Work out the finished part from the listing and answer in its coordinate system (mm). Round coordinates to 2 decimals unless told otherwise and drop trailing zeros. Order: outer loops, then holes, each group sorted by start corner. A loop starts at its lowest first (then second) coordinate and runs counter-clockwise, first axis right, second up. Notation, with made-up numbers: (26.5, 30) - (63.5, 30) arc R22 ccw to (63.5, 64) - close; hole circle Ø1 at (-3, -36.75). An arc over 180 degrees is marked (long way). Answer in a Markdown table with one row per item.
from build123d import *

# Parameters (mm, degrees)
BOSS_EXTRUDE1_DEPTH      = 39.6875
SKETCH2_R                = 1.4351
CUT_EXTRUDE1_DEPTH       = 42.03119412
F_5_16_24_TAPPED_HOLE1_D = 6.9088


with BuildPart() as part:
    # Sketch1 → Boss-Extrude1 (new body)
    with BuildSketch(Plane.XY):
        Polygon((0, 0), (9.9187, 0), (6.7437, -3.175), (0, -3.175), align=None)
    extrude(amount=BOSS_EXTRUDE1_DEPTH)

    # Mirror1: part across plane


with BuildPart() as part_1:
    add(part.part)
    add(part.part.mirror(Plane(origin=(0, -3.175, 39.6875), x_dir=(0, 0, 1), z_dir=(1, 0, 0))))

    # Sketch2 → Cut-Extrude1 (cut, through all)
    with BuildSketch(Plane(origin=(0, 0, 0), x_dir=(1, 0, 0), z_dir=(0, 1, 0))):
        with Locations(Location((0, -36.5125, 0), (0, 0, 180))):
            Circle(SKETCH2_R)
    extrude(amount=-CUT_EXTRUDE1_DEPTH, mode=Mode.SUBTRACT)

    # Mirror2: part across plane


with BuildPart() as part_2:
    add(part_1.part)
    add(part_1.part.mirror(Plane(origin=(0, 0, 0), x_dir=(1, 0, 0), z_dir=(0, 0, -1))))

    # 5/16-24 Tapped Hole1 (through all)
    with Locations(Plane(origin=(0, 0, 0), x_dir=(-1, 0, 0), z_dir=(0, 1, 0))):
        with Locations((0, 0)):
            Hole(F_5_16_24_TAPPED_HOLE1_D / 2)


solid = part_2.part
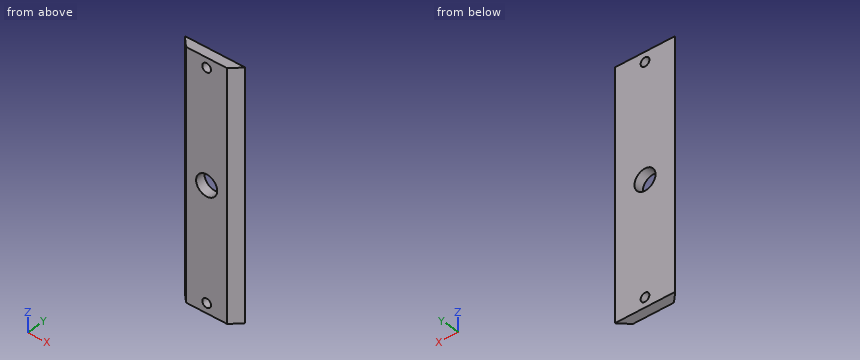
1) Find section A-A, the plane x = 0. Give the vertices of the cut face in (y, z) (1 decimal).
Filled in:
| item | result |
|---|---|
| outline | (-3.2, -39.7) - (0, -39.7) - (0, -37.9) - (-3.2, -37.9) - close; (-3.2, -35.1) - (0, -35.1) - (0, -3.5) - (-3.2, -3.5) - close; (-3.2, 3.5) - (0, 3.5) - (0, 35.1) - (-3.2, 35.1) - close; (-3.2, 37.9) - (0, 37.9) - (0, 39.7) - (-3.2, 39.7) - close |
2) Find section B-B, the plane z = 0. Give the vertices of the cut face in (x, y) (3 decimals), then the cut area to 3 significant figures.
Filled in:
| item | result |
|---|---|
| outline | (-9.919, 0) - (-6.744, -3.175) - (-3.454, -3.175) - (-3.454, 0) - close; (3.454, -3.175) - (6.744, -3.175) - (9.919, 0) - (3.454, 0) - close |
| area | 31.0 mm^2 |
3) Each of these flat-tipped pins is pushed along its axis until it touches: pin 1 (1 mm diameter, centred on x = 7.5, z = -28, fed in from -Y); pin 2 (2.5 mm diameter, centred on x = 0, z = 36.51, fed in from +Y). Where does it stop, or does it pass through?
Filled in:
| item | result |
|---|---|
| pin 1 | stops at y = -2.92 |
| pin 2 | passes through |
4) Find section D-D, the plane z = -27.5. Give the vertices of the cut face in (x, y) (3 decimals).
Filled in:
| item | result |
|---|---|
| outline | (-9.919, 0) - (-6.744, -3.175) - (6.744, -3.175) - (9.919, 0) - close |
5) Find the intervals of material crossed by probe 1 along Z at (x, y) = (0, -1.1); probe 2 along Z at (x, y) = (1.25, -1.6); probe 3 along Z at (x, y) = (-2.75, -2.3), in increasing order. Write a range as from..to.
Filled in:
| item | result |
|---|---|
| probe 1 | z = -39.69..-37.95, -35.08..-3.45, 3.45..35.08, 37.95..39.69 |
| probe 2 | z = -39.69..-37.22, -35.81..-3.22, 3.22..35.81, 37.22..39.69 |
| probe 3 | z = -39.69..-2.09, 2.09..39.69 |
6) Find section C-C, the plane y = -1. Give the vertices of the cut face in (x, z), then the cut area to 3 significant figures.
Filled in:
| item | result |
|---|---|
| outline | (-8.92, -39.69) - (8.92, -39.69) - (8.92, 39.69) - (-8.92, 39.69) - close; hole circle Ø6.91 at (0, 0); hole circle Ø2.87 at (0, -36.51); hole circle Ø2.87 at (0, 36.51) |
| area | 1,370 mm^2 |
